Part model, mm, in its own coordinate system. Face numbers are marked on the shaded views. A direction names the side the tool comes from. Give positions to 0.01 mm unless a question says otherwise; leave off trailing zeros. Order: outer loops, then holes, each group sorted by start corner. A loop starts at its lowest first (then second) coordinate and runs counter-clockwise, first axis right, second up. Notation, with made-up numbers: (-28.75, 49) -> (28.25, 49) arc R18 ccw to (28.25, 53) -> close; hole circle Ø1 at (46.25, 7). An arc over 180 degrees is marked (long way). Write item = value, one per line. Start each with the question number.
Item 1: Tool access for the marked faces 4 and 5: list every direction of +Z, -Z, +X, -X, +Y, -Y with a clear straight run to the whole face (end or side of a thin tool).
Item 2: Band-saw the part on D-D on x = 55. Write the cut outline in (y, z).
Item 3: Band-saw the part on B-B on y = -11.5. Write the cut outline in (x, z), plus the area to 3 significant figures.
Item 4: Pull direction X, two halves, no side cores. Call the marked faces 1, 2 and 3: +X half, -X half, draft (parallel to the pull), parting line (faces both ways), or undercut.
Item 5: Flat gauge pins, fed straight in: P1, Ø0.5, axis at y = -26.5, z = 19, coming from the -X side; P2, Ø3, axis at x = 35.5, y = -14.5, coming from the +Z side; P3, Ø1, axis at x = 61.5, y = -6.5, coming from the -Z side. Where does each tip first touch, or does it go through?
Item 6: Drill centre lines: line 1 along Y through (x, z) = (25.5, -7); line 2 along X through (y, z) = (-3.25, 6); line 3 along Z through (x, y) = (27, -9.5). Where is each one in solid material? Low to high.
Item 7: Band-saw the part on C-C on z = 3.5. Write the cut outline in (x, y).
Item 8: Band-saw the part on A-A on x = 43.5. Write the cut outline in (y, z).
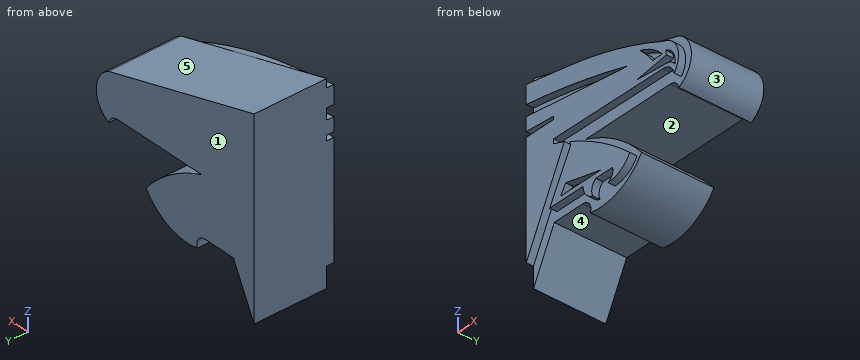
```python
from build123d import *

# Parameters (mm, degrees)
F1_DEPTH = 25.4
F3_DEPTH = 2.54


with BuildPart() as f1:
    # F0 (on Front) → F1 (new body)
    with BuildSketch(Plane.XZ):
        with BuildLine():
            Line((4.675265, 38.648338), (4.675265, -29.022353))
            Line((4.675265, -29.022353), (13.136835, -12.086689))
            Line((13.136835, -12.086689), (24.644025, -12.086689))
            ThreePointArc((24.644025, -12.086689), (27.390181, -13.518342), (27.788887, -16.589504))
            ThreePointArc((27.788887, -16.589504), (39.534536, -15.492547), (48.578784, -7.918567))
            ThreePointArc((48.578784, -7.918567), (38.344977, 1.625304), (25.908433, 8.040027))
            Line((25.908433, 8.040027), (60.161997, 8.040027))
            ThreePointArc((60.161997, 8.040027), (62.441504, 7.233012), (63.705467, 5.171502))
            ThreePointArc((63.705467, 5.171502), (68.823481, 13.439604), (63.705467, 21.707706))
            Line((63.705467, 21.707706), (4.675265, 38.648338))
        make_face()
    extrude(amount=F1_DEPTH)

    # F2 (on face) → F3 (join)
    with BuildSketch(Plane.XZ.offset(25.4)):
        with BuildLine():
            ThreePointArc((4.675265, 29.146321), (25.516102, 25.450284), (46.005655, 20.141857))
            ThreePointArc((46.005655, 20.141857), (25.329763, 22.617176), (4.675265, 25.265086))
            Line((4.675265, 25.265086), (4.675265, 20.410509))
            Line((4.675265, 20.410509), (15.810639, 19.637108))
            Line((15.810639, 19.637108), (15.810639, 18.545922))
            Line((15.810639, 18.545922), (4.675265, 18.545922))
            Line((4.675265, 18.545922), (4.675265, -21.817246))
            Line((4.675265, -21.817246), (20.169701, 9.19456))
            Line((20.169701, 9.19456), (15.810639, 10.708986))
            Line((15.810639, 10.708986), (15.810639, 12.321869))
            Line((15.810639, 12.321869), (60.161997, 11.876815))
            ThreePointArc((60.161997, 11.876815), (63.147761, 10.778846), (64.766154, 8.040027))
            ThreePointArc((64.766154, 8.040027), (66.027213, 15.656968), (60.161997, 20.677656))
            ThreePointArc((60.161997, 20.677656), (41.195878, 27.981513), (21.435434, 32.733861))
            Line((21.435434, 32.733861), (4.675265, 35.614753))
            Line((4.675265, 35.614753), (4.675265, 29.146321))
        make_face()
        with BuildLine():
            Line((61.803415, 12.841351), (49.711283, 13.763633))
            Line((49.711283, 13.763633), (61.598465, 15.608195))
            Line((61.598465, 15.608195), (61.341725, 17.26274))
            ThreePointArc((61.341725, 17.26274), (64.422395, 14.726928), (65.082639, 10.791837))
            ThreePointArc((65.082639, 10.791837), (63.695147, 12.219986), (61.803415, 12.841351))
        make_face(mode=Mode.SUBTRACT)
        with BuildLine():
            Line((59.874482, 16.794579), (56.074578, 16.587311))
            ThreePointArc((56.074578, 16.587311), (53.621941, 19.743599), (50.823804, 22.598071))
            ThreePointArc((50.823804, 22.598071), (55.773558, 20.35821), (59.874482, 16.794579))
        make_face(mode=Mode.SUBTRACT)
        with BuildLine():
            Line((22.387989, 8.040027), (22.718249, 6.635162))
            Line((22.718249, 6.635162), (14.179533, -9.200274))
            Line((14.179533, -9.200274), (27.788887, -9.200274))
            ThreePointArc((27.788887, -9.200274), (28.86277, -12.447594), (31.722713, -14.323504))
            ThreePointArc((31.722713, -14.323504), (31.380156, -11.560312), (32.983219, -9.283744))
            Line((32.983219, -9.283744), (39.701112, -9.283744))
            ThreePointArc((39.701112, -9.283744), (39.55028, -11.611776), (37.866078, -13.22607))
            ThreePointArc((37.866078, -13.22607), (42.999226, -11.895955), (46.722099, -8.119896))
            ThreePointArc((46.722099, -8.119896), (35.211974, 0.949291), (22.387989, 8.040027))
        make_face()
        Polygon((18.681765, -7.64778), (20.700006, -4.387544), (34.982949, -7.64778), align=None, mode=Mode.SUBTRACT)
    extrude(amount=F3_DEPTH)


solid = f1.part
```
Values found:
q1.face_4 = -Z, +Y, -Y
q1.face_5 = +Z, +X, +Y, -Y
q2.outline = (-27.94, 11.93) -> (-25.4, 11.93) -> (-25.4, 8.04) -> (0, 8.04) -> (0, 24.21) -> (-25.4, 24.21) -> (-25.4, 22.95) -> (-27.94, 22.95) -> (-27.94, 20.83) -> (-25.4, 20.83) -> (-25.4, 18.06) -> (-27.94, 18.06) -> (-27.94, 14.58) -> (-25.4, 14.58) -> (-25.4, 13.36) -> (-27.94, 13.36) -> close
q3.outline = (4.68, -29.02) -> (13.14, -12.09) -> (24.64, -12.09) arc R3.35 cw to (27.79, -16.59) arc R19.83 ccw to (48.58, -7.92) arc R51.17 ccw to (25.91, 8.04) -> (60.16, 8.04) arc R3.62 cw to (63.71, 5.17) arc R9.24 ccw to (63.71, 21.71) -> (4.68, 38.65) -> close
q3.area = 2,240 mm^2
q4.face_1 = draft
q4.face_2 = undercut
q4.face_3 = +X half
q5.P1 = 15.81
q5.P2 = 30.23
q5.P3 = 7.54
q6.line_1 = -25.4 to 0
q6.line_2 = 4.68 to 30.85, 63.42 to 65.06
q6.line_3 = -13.06 to 7.64, 8.04 to 32.24
q7.outline = (4.68, -27.94) -> (17.32, -27.94) -> (17.32, -25.4) -> (21.03, -25.4) -> (21.03, -27.94) -> (31.14, -27.94) -> (31.14, -25.4) -> (35.48, -25.4) -> (35.48, 0) -> (4.68, 0) -> close
q8.outline = (-27.94, -11.59) -> (-25.4, -11.59) -> (-25.4, -13.27) -> (0, -13.27) -> (0, -2.53) -> (-25.4, -2.53) -> (-25.4, -5.27) -> (-27.94, -5.27) -> close; (-27.94, 12.04) -> (-25.4, 12.04) -> (-25.4, 8.04) -> (0, 8.04) -> (0, 27.51) -> (-25.4, 27.51) -> (-25.4, 27.24) -> (-27.94, 27.24) -> (-27.94, 20.88) -> (-25.4, 20.88) -> (-25.4, 20.43) -> (-27.94, 20.43) -> close
